Source: CAD feature listing. Evaluate the final solid. Frame: model axes, mm. A direction names the side the tool comes from. Give positions to 0.01 mm unless a question says otherwise; leave off trailing zeros. Return JSON: item names as keys, results as strings. Group by question number.
(1) Access query for faces 4 (the face through (3.65, 0, -1)), 5 (the face through (0, 3.65, -1)), 6 (the face through (0, -3.65, -1)), 7 (the face through (-6, -10, -1)), 8 (the face through (-10, -6, -1)). Directions: +Z, -Z, +X, -X, +Y, -Y. A direction counts if a zero-diameter tool reaches every point of the face in a straight line with its end or side. Return the directions, or none.
(2) Draft query along X for faces 1 (the face through (-3.65, 0, -1)), 2 (the face through (-0.1, 2.4, 100)), 3 (the face through (-2.15, -0.09, -1.4)). Return one class per face: released by +X, released by -X, zero draft, split by the parting line, or undercut.
(3) Pin query (flat end, axial travel): pin 1 (1 mm diameter, centred on y = -2.5, z = 70, fed in from +X); pin 2 (0.5 mm diameter, centred on y = -9, z = 31.5, fed in from +X); pin 3 (3.5 mm diameter, centred on x = 0.5, z = 47.5, fed in from +Y). Return the tip coordinate at first contact, or that it passes through.
(4) Ray query, line 1 (Y direction, x = 4, z = -39); line 2 (X direction, y = 0.25, z = 62); line 3 (Y direction, x = 0, z = -18). Return the intervals inside material, ascending. Write a range as from..to.
Autodesk Inventor part; units mm, degrees
ref_plane "YZ Plane" through (0, 0, 0) normal (1, 0, 0) x (0, 1, 0)
ref_plane "XZ Plane" through (0, 0, 0) normal (0, 1, 0) x (-1, 0, 0)
ref_plane "XY Plane" through (0, 0, 0) normal (0, 0, 1) x (1, 0, 0)
sketch "Sketch1" plane through (0, 0, 0) normal (0, 0, 1) x (1, 0, 0)
  circle A0 centre (0, 0) radius 2.15
  line L0 (-10, 10) -> (-2.5, 10)
  line L1 (-2.5, 10) -> (-2.5, 8.2)
  line L2 (-2.5, 8.2) -> (-6.9272, 8.2)
  line L3 (-6.9272, 8.2) -> (-2.3772, 3.65)
  line L4 (-2.3772, 3.65) -> (2.3772, 3.65)
  line L5 (2.3772, 3.65) -> (6.9272, 8.2)
  line L6 (6.9272, 8.2) -> (2.5, 8.2)
  line L7 (2.5, 8.2) -> (2.5, 10)
  line L8 (2.5, 10) -> (10, 10)
  line L9 (10, 10) -> (10, 2.5)
  line L10 (10, 2.5) -> (8.2, 2.5)
  line L11 (8.2, 2.5) -> (8.2, 6.9272)
  line L12 (8.2, 6.9272) -> (3.65, 2.3772)
  line L13 (3.65, 2.3772) -> (3.65, -2.3772)
  line L14 (3.65, -2.3772) -> (8.2, -6.9272)
  line L15 (8.2, -6.9272) -> (8.2, -2.5)
  line L16 (8.2, -2.5) -> (10, -2.5)
  line L17 (10, -2.5) -> (10, -10)
  line L18 (10, -10) -> (2.5, -10)
  line L19 (2.5, -10) -> (2.5, -8.2)
  line L20 (2.5, -8.2) -> (6.9272, -8.2)
  line L21 (6.9272, -8.2) -> (2.3772, -3.65)
  line L22 (2.3772, -3.65) -> (-2.3772, -3.65)
  line L23 (-2.3772, -3.65) -> (-6.9272, -8.2)
  line L24 (-6.9272, -8.2) -> (-2.5, -8.2)
  line L25 (-2.5, -8.2) -> (-2.5, -10)
  line L26 (-2.5, -10) -> (-10, -10)
  line L27 (-10, -10) -> (-10, -2.5)
  line L28 (-10, -2.5) -> (-8.2, -2.5)
  line L29 (-8.2, -2.5) -> (-8.2, -6.9272)
  line L30 (-8.2, -6.9272) -> (-3.65, -2.3772)
  line L31 (-3.65, -2.3772) -> (-3.65, 2.3772)
  line L32 (-3.65, 2.3772) -> (-8.2, 6.9272)
  line L33 (-8.2, 6.9272) -> (-8.2, 2.5)
  line L34 (-8.2, 2.5) -> (-10, 2.5)
  line L35 (-10, 2.5) -> (-10, 10)
  line L36 (0, 0) -> (-30.8654, 30.8654)
  line L37 (0, 0) -> (30.8654, 30.8654)
  line L38 (0, 0) -> (42.5392, 0)
  line L39 (0, 0) -> (0, 44.3419)
  dimension "d0" = 45
  dimension "d1" = 90
  dimension "Breite" = 20
  dimension "Tiefe_Schiene" = 6.35
  dimension "d2" = 1.8
  dimension "Durchmesser_Loch" = 4.3
  dimension "Wandstaerke" = 1.8
  dimension "d3" = 1.8
  dimension "Breite_Schiene" = 5
  dimension "d4" = 5
extrude "Extrusion1" add sketch "Sketch1" along normal mid plane 200 contours L38 L13 L14 L15 L16 L17 L18 L19 L20 L21 L22 L23 L24 L25 L26 L27 L28 L29 L30 L31 L32 L33 L34 L35 L36 A0 | A0 L37 L9 L10 L11 L12 L13 L38 | A0 L39 L4 L5 L6 L7 L8 L37 | L36 L0 L1 L2 L3 L4 L39 A0
fillet "Fillet1" radius 2 4 edges at (10, 10, 0) (-10, 10, 0) (10, -10, 0) (-10, -10, 0)
fillet "Fillet2" radius 0.2 8 edges at (-2.5, 8.2, 0) (2.5, 8.2, 0) (8.2, 2.5, 0) (8.2, -2.5, 0) (-2.5, -8.2, 0) (-8.2, -2.5, 0) (-8.2, 2.5, 0) (2.5, -8.2, 0)
fillet "Fillet3" radius 0.7 16 edges at (-2.5, 10, 0) (2.5, 10, 0) (10, 2.5, 0) (10, -2.5, 0) (2.5, -10, 0) (-2.5, -10, 0) (-10, -2.5, 0) (-10, 2.5, 0) (-6.9272, -8.2, 0) (-8.2, -6.9272, 0) (6.9272, -8.2, 0) (8.2, -6.9272, 0) (8.2, 6.9272, 0) (6.9272, 8.2, 0) (-6.9272, 8.2, 0) (-8.2, 6.9272, 0)
fillet "Fillet4" radius 2 8 edges at (-3.65, 2.3772, 0) (-2.3772, 3.65, 0) (2.3772, 3.65, 0) (3.65, 2.3772, 0) (3.65, -2.3772, 0) (2.3772, -3.65, 0) (-2.3772, -3.65, 0) (-3.65, -2.3772, 0)
equation "\"d2\" = Wandstaerke"
equation "\"d3\" = Wandstaerke"
equation "\"d4\" = Breite_Schiene"
properties part number "503.025.01_ITEM_20x20_200mm"
Answers:
{
 "1": {"face 4": "+Z, -Z, +X", "face 5": "+Z, -Z, +Y", "face 6": "+Z, -Z, -Y", "face 7": "+Z, -Z, +X, -X, -Y", "face 8": "+Z, -Z, -X, +Y, -Y"},
 "2": {"face 1": "released by -X", "face 2": "zero draft", "face 3": "undercut"},
 "3": {"pin 1": "x = 9.97", "pin 2": "x = 9.85", "pin 3": "y = 3.78"},
 "4": {"line 1": "-10..-8.2, -5.27..-2.68, 2.68..5.27, 8.2..10", "line 2": "-3.65..-2.14, 2.14..3.65", "line 3": "-3.65..-2.15, 2.15..3.65"}
}
